from build123d import *

# Parameters (mm, degrees)
SKETCH_1_R          = 25
SKETCH_1_R_2        = 1.525
SKETCH_1_R_3        = 10
EXTRUDE_1_DEPTH     = 3
EXTRUDE_2_DEPTH     = 3
FILLET_1_R          = 3
SKETCH_4_R          = 1.515
CUT_EXTRUDE_1_DEPTH = 10


with BuildPart() as part:
    # 草图1 → 凸台-拉伸1 (new body)
    with BuildSketch(Plane.XY):
        Circle(SKETCH_1_R)
        with Locations((0, 20)):
            Circle(SKETCH_1_R_2, mode=Mode.SUBTRACT)
        with Locations((17.320508076, 10)):
            Circle(SKETCH_1_R_2, mode=Mode.SUBTRACT)
        with Locations((17.320508076, -10)):
            Circle(SKETCH_1_R_2, mode=Mode.SUBTRACT)
        with Locations((0, -20)):
            Circle(SKETCH_1_R_2, mode=Mode.SUBTRACT)
        Circle(SKETCH_1_R_3, mode=Mode.SUBTRACT)
        with Locations((-17.320508076, -10)):
            Circle(SKETCH_1_R_2, mode=Mode.SUBTRACT)
        with Locations((-17.320508076, 10)):
            Circle(SKETCH_1_R_2, mode=Mode.SUBTRACT)
    extrude(amount=EXTRUDE_1_DEPTH)

    # 草图3 → 凸台-拉伸2 (add)
    with BuildSketch(Plane.XY.offset(3)):
        with BuildLine():
            Line((15, 20), (40, 20))
            Line((40, 20), (40, -20))
            Line((40, -20), (15, -20))
            ThreePointArc((15, -20), (25, 0), (15, 20))
        make_face()
        with BuildLine():
            Line((-40, -20), (-15, -20))
            ThreePointArc((-15, -20), (-25, 0), (-15, 20))
            Line((-15, 20), (-40, 20))
            Line((-40, 20), (-40, -20))
        make_face()
    extrude(amount=-EXTRUDE_2_DEPTH)

    # 圆角1
    fillet_1_edges = [part.edges().sort_by_distance(p)[0] for p in [
        (40, 20, 1.5),
        (40, -20, 1.5),
        (15, -20, 1.5),
        (15, 20, 1.5),
        (-40, -20, 1.5),
        (-40, 20, 1.5),
        (-15, 20, 1.5),
        (-15, -20, 1.5),
    ]]
    fillet(fillet_1_edges, radius=FILLET_1_R)

    # 草图4 → 切除-拉伸1 (cut)
    with BuildSketch(Plane.XY.offset(3)):
        with Locations((-34, 15)):
            Circle(SKETCH_4_R)
        with Locations((-34, -5)):
            Circle(SKETCH_4_R)
        with Locations((34, -5)):
            Circle(SKETCH_4_R)
        with Locations((34, 15)):
            Circle(SKETCH_4_R)
    extrude(amount=-CUT_EXTRUDE_1_DEPTH, mode=Mode.SUBTRACT)


solid = part.part
Can you work these out from the model? Positions are in its coordinate system, mm. A direction names the side the tool comes from. Coordinates: 2 decimals unless noted, no trailing zeros. Order: outer loops, then holes, each group sorted by start corner. A loop starts at its lowest first (then second) coordinate and runs counter-clockwise, first axis right, second up. Notation, with made-up numbers: (87.25, -39) - (105.25, -39) arc R19 ccw to (105.25, -13) - close; hole circle Ø1 at (6.5, 42.25). An arc over 180 degrees is marked (long way). Answer as a JSON object with one key per item and string values. Group by question number.
Q1. On a 3-axis mill with a long thin cutter (end or side, diameter ignored), from which of +Z, -Z, +X, -X, +Y, -Y can I reach the whole of each face in a straight line? I mean faces 4 (the face through (0, 25, 1)), 5 (the face through (-26, 20, 2)), 6 (the face through (-27, -20, 2)). Say none if no direction works.
Q2. Will these pins go through, and if not, where does the flat tip stop? P1, Ø1.5, axis at x = -17.5, z = 2.5, coming from the +Y side; P2, Ø5, axis at x = 17.32, y = -10, coming from the +Z side.
Q3. Imagine slicing it at D-D (x = -7). Please give me the cut outline in (y, z).
Q4. Imagine slicing it at C-C (z = 0.95). Give the number of separate pieces and of enclosed holes in the cut face, and give its area (3 significant figures).
Q5. Imagine slicing it at B-B (y = 15). Please give me the cut outline in (x, z) (3 decimals).
Q6. Imagine slicing it at A-A (y = 0). Please give me the cut outline in (x, z), and give its area (3 significant figures).
Q7. We'd pull the mould along X, two halves only. Please class faces 1 (the face through (0, -25, 1)), 2 (the face through (9, 6, 0)), 3 (the face through (18.14, 11.286, 1.479)): +X half, -X half, draft (parallel to the pull), parting line (faces both ways), or undercut.
Q8. I need wall thicknesses on line 1 (Y direction, x = 0, z = 1.5) (3 decimals); line 2 (Y direction, x = 34, z = 2.75) (3 decimals); line 3 (Y direction, x = 34.5, z = 2.5). Which ranges of each line are inside material? Lowest first, please. Write a range as from..to.
Determined:
{
 "1": {"face 4": "+Z, -Z, +Y", "face 5": "+Z, -Z, -X, +Y", "face 6": "+Z, -Z, -X, -Y"},
 "2": {"P1": "stops at y = 20", "P2": "stops at z = 3"},
 "3": {"outline": "(-24, 0) - (-7.14, 0) - (-7.14, 3) - (-24, 3) - close; (7.14, 0) - (24, 0) - (24, 3) - (7.14, 3) - close"},
 "4": {"separate pieces": "1", "enclosed holes": "11", "area": "3,010 mm2"},
 "5": {"outline": "(-40, 0) - (-35.515, 0) - (-35.515, 3) - (-40, 3) - close; (-32.485, 0) - (32.485, 0) - (32.485, 3) - (-32.485, 3) - close; (35.515, 0) - (40, 0) - (40, 3) - (35.515, 3) - close"},
 "6": {"outline": "(-40, 0) - (-10, 0) - (-10, 3) - (-40, 3) - close; (10, 0) - (40, 0) - (40, 3) - (10, 3) - close", "area": "180 mm2"},
 "7": {"face 1": "parting line", "face 2": "draft", "face 3": "undercut"},
 "8": {"line 1": "y = -25..-21.525, -18.475..-10, 10..18.475, 21.525..25", "line 2": "y = -20..-6.515, -3.485..13.485, 16.515..20", "line 3": "y = -20..-6.43, -3.57..13.57, 16.43..20"}
}
